Design review of the part built by this model. Coordinates are the model's own, in mm. Face numbers are marked on the shaded views. Coordinates: 2 decimals unless noted, no trailing zeros. Loops run counter-clockwise (first coordinate to the right, second up) from the corner with the lowest first, then second, coordinate; pieces in that order, holes last. Notation, with made-up numbers: (78, 71.5) - (83, 71.5) arc R18 cw to (83, 85.5) - close; hole circle Ø5 at (-10, 6.5). An arc over 180 degrees is marked (long way). Use one line per item in the form item = value. Start each with the question number.
(1) Add section D-D (y = 0.3). State the section outline as (x, z) points.
(2) The part is to be moulded in two halves that separate along Z. For the marked faces 1, 2 and 3, say which applies: pulls with the +Z half, pulls with the -Z half, needs draft (parallel to the pull), parting line crosses it, or undercut.
(3) Add section A-A (x = 0). State the section outline as (y, z) points.
(4) For L1, parallel to X at y = 1.55, z = -0.75; L2, parallel to X at y = 1, z = 0; L3, parallel to Z at x = -15, y = 1.45, list the stretches that pass through material, from the lowest coordinate up.
(5) Add section B-B (z = 0). State the section outline as (x, y) points.
(6) Add section C-C (x = -15). State the section outline as (y, z) points, plus the area to 3 significant figures.
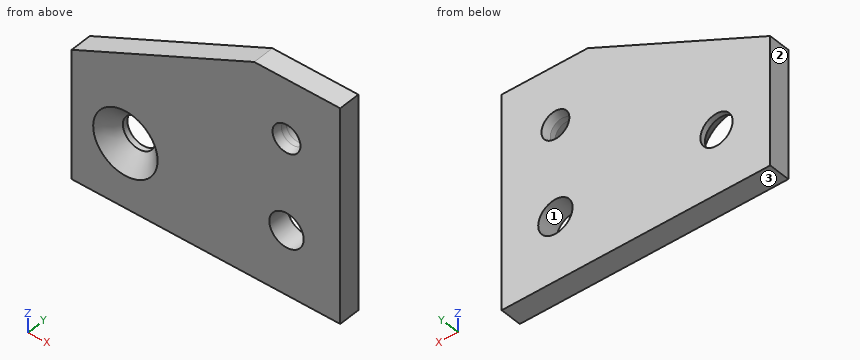
```python
from build123d import *

# Parameters (mm, degrees)
SKETCH1_R             = 1.6
SKETCH1_R_2           = 1.5
SKETCH1_R_3           = 1.1
EXTRUDE1_DEPTH        = 2
CHAMFER1_SIZE         = 1.5
CHAMFER2_SIZE         = 0.2
CHAMFER2_SIZE2        = 0.746410162
CHAMFER2_PART_2_SIZE  = 0.2
CHAMFER2_PART_2_SIZE2 = 0.746410162


with BuildPart() as part:
    # Sketch1 → Extrude1 (new body)
    with BuildSketch(Plane(origin=(0, 0, 0), x_dir=(1, 0, 0), z_dir=(0, 1, 0))):
        Polygon((-20, 6), (5, 6), (5, -14), (-3, -14), (-20, -6), align=None)
        with Locations(Location((0, 0, 0), (0, 0, 270))):  # turned: the seam where the file's is
            Circle(SKETCH1_R, mode=Mode.SUBTRACT)
        with Locations(Location((-15, 0, 0), (0, 0, 270))):  # turned: the seam where the file's is
            Circle(SKETCH1_R_2, mode=Mode.SUBTRACT)
        with Locations(Location((0, -8.5, 0), (0, 0, 270))):  # turned: the seam where the file's is
            Circle(SKETCH1_R_3, mode=Mode.SUBTRACT)
    extrude(amount=EXTRUDE1_DEPTH)

    # Chamfer1
    chamfer1_edges = [part.edges().sort_by_distance(p)[0] for p in [
        (-15, 0, -1.5),
    ]]
    chamfer(chamfer1_edges, length=CHAMFER1_SIZE)

    # Chamfer2
    chamfer2_edges = [part.edges().sort_by_distance(p)[0] for p in [
        (0, 0, 7.4),
    ]]
    chamfer2_side = [part.faces().sort_by_distance(p)[0] for p in [
        (-5.999814113, 0, 3.054548244),
    ]]
    chamfer(chamfer2_edges, length=CHAMFER2_SIZE, length2=CHAMFER2_SIZE2, reference=chamfer2_side[0])

    # Chamfer2 part 2
    chamfer2_part_2_edges = [part.edges().sort_by_distance(p)[0] for p in [
        (0, 2, 7.4),
    ]]
    chamfer2_part_2_side = [part.faces().sort_by_distance(p)[0] for p in [
        (-6.46183643, 2, 2.897743765),
    ]]
    chamfer(chamfer2_part_2_edges, length=CHAMFER2_PART_2_SIZE, length2=CHAMFER2_PART_2_SIZE2, reference=chamfer2_part_2_side[0])


solid = part.part
```
Computed values:
q1.outline = (-20, -6) - (5, -6) - (5, 14) - (-3, 14) - (-20, 6) - close; hole circle Ø5.4 at (-15, 0); hole circle Ø3.2 at (0, 0); hole circle Ø2.44 at (0, 8.5)
q2.face_1 = undercut
q2.face_2 = needs draft
q2.face_3 = pulls with the -Z half
q3.outline = (0, -6) - (2, -6) - (2, -1.6) - (0, -1.6) - close; (0, 1.6) - (2, 1.6) - (2, 7.2) - (1.25, 7.4) - (0.75, 7.4) - (0, 7.2) - close; (0, 9.8) - (0.75, 9.6) - (1.25, 9.6) - (2, 9.8) - (2, 14) - (0, 14) - close
q4.L1 = -20 to -16.3, -13.7 to -1.41, 1.41 to 5
q4.L2 = -20 to -17, -13 to -1.6, 1.6 to 5
q4.L3 = -6 to -1.55, 1.55 to 8.35
q5.outline = (-20, 0) - (-18, 0) - (-16.5, 1.5) - (-16.5, 2) - (-20, 2) - close; (-13.5, 1.5) - (-12, 0) - (-1.6, 0) - (-1.6, 2) - (-13.5, 2) - close; (1.6, 0) - (5, 0) - (5, 2) - (1.6, 2) - close
q6.outline = (0, -6) - (2, -6) - (2, -1.5) - (1.5, -1.5) - (0, -3) - close; (0, 3) - (1.5, 1.5) - (2, 1.5) - (2, 8.35) - (0, 8.35) - close
q6.area = 20.5 mm^2
